The listing builds one solid part. Answer for the finished solid, in the listing's coordinates (mm). Give positions to 0.01 mm unless a question says otherwise; leave off trailing zeros. Write each loop counter-clockwise with the first axis right and the second up, starting at its lowest first coordinate (ties: lowest second). Pieces come first, ordered by that corner, then holes. Notation, with made-up numbers: (-10.75, -27) - (19.25, -27) arc R12 cw to (19.25, -9) - close; hole circle Ø11 at (-1, 71). An arc over 180 degrees is marked (long way). One line per item, written item: value. Start each with the question number.
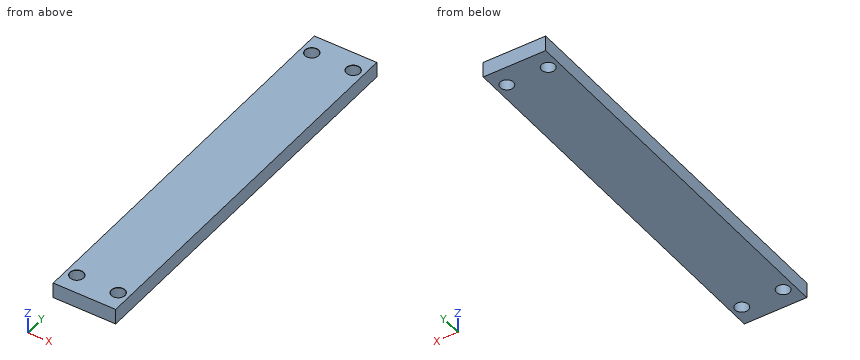
from build123d import *

# Parameters (mm, degrees)
CROQUIS1_W                               = 8
CROQUIS1_H                               = 50
SALIENTE_EXTRUIR1_DEPTH                  = 2
TALADRO_DE_MARGEN_PARA_M1_61_D           = 1.7
TALADRO_DE_MARGEN_PARA_M1_61_CSINK_D     = 1.75
TALADRO_DE_MARGEN_PARA_M1_61_CSINK_ANGLE = 82
TALADRO_DE_MARGEN_PARA_M1_62_D           = 1.7
TALADRO_DE_MARGEN_PARA_M1_62_CSINK_D     = 1.75
TALADRO_DE_MARGEN_PARA_M1_62_CSINK_ANGLE = 82


with BuildPart() as part:
    # Croquis1 → Saliente-Extruir1 (new body)
    with BuildSketch(Plane.XY):
        with Locations((4, 25)):
            Rectangle(CROQUIS1_W, CROQUIS1_H)
    extrude(amount=SALIENTE_EXTRUIR1_DEPTH)

    # Taladro de margen para M1.61 (through all)
    with Locations(Plane.XY.offset(2)):
        with Locations((1.35, 47.5), (6.65, 47.5)):
            CounterSinkHole(TALADRO_DE_MARGEN_PARA_M1_61_D / 2, TALADRO_DE_MARGEN_PARA_M1_61_CSINK_D / 2, counter_sink_angle=TALADRO_DE_MARGEN_PARA_M1_61_CSINK_ANGLE)

    # Taladro de margen para M1.62 (through all)
    with Locations(Plane.XY.offset(2)):
        with Locations((1.35, 2.5), (6.65, 2.5)):
            CounterSinkHole(TALADRO_DE_MARGEN_PARA_M1_62_D / 2, TALADRO_DE_MARGEN_PARA_M1_62_CSINK_D / 2, counter_sink_angle=TALADRO_DE_MARGEN_PARA_M1_62_CSINK_ANGLE)


solid = part.part
Item 1: Find section B-B on y = 47.5. Determine the outline of the cut face in (x, z) (3 decimals), plus the area to 3 significant figures.
Item 2: Straight lines are drawn through the part: line 1 along Y through (x, z) = (1.35, 1.2); line 2 along X through (y, z) = (47.5, 0.8); line 3 along Y through (x, z) = (0.75, 0.1). For each, find the intervals that lie inside material, in ascending order.
Item 3: Find section C-C on z = 0.45. Determine the outline of the cut face in (x, y), plus the area to 3 significant figures.
Item 4: Find section A-A on x = 1.35. Determine the outline of the cut face in (y, z) (3 decimals).
Values:
1. outline: (0, 0) - (0.5, 0) - (0.5, 1.971) - (0.475, 2) - (0, 2) - close; (2.2, 0) - (5.8, 0) - (5.8, 1.971) - (5.775, 2) - (2.225, 2) - (2.2, 1.971) - close; (7.5, 0) - (8, 0) - (8, 2) - (7.525, 2) - (7.5, 1.971) - close
1. area: 9.20 mm^2
2. line 1: 0 to 1.65, 3.35 to 46.65, 48.35 to 50
2. line 2: 0 to 0.5, 2.2 to 5.8, 7.5 to 8
2. line 3: 0 to 1.9, 3.1 to 46.9, 48.1 to 50
3. outline: (0, 0) - (8, 0) - (8, 50) - (0, 50) - close; hole circle Ø1.7 at (1.35, 2.5); hole circle Ø1.7 at (1.35, 47.5); hole circle Ø1.7 at (6.65, 2.5); hole circle Ø1.7 at (6.65, 47.5)
3. area: 391 mm^2
4. outline: (0, 0) - (1.65, 0) - (1.65, 1.971) - (1.625, 2) - (0, 2) - close; (3.35, 0) - (46.65, 0) - (46.65, 1.971) - (46.625, 2) - (3.375, 2) - (3.35, 1.971) - close; (48.35, 0) - (50, 0) - (50, 2) - (48.375, 2) - (48.35, 1.971) - close
